Can you work these out from the model? Positions are in its coordinate system, mm. A direction names the side the tool comes from. Give positions to 0.01 mm unless a question says otherwise; leave off trailing zeros. Loops run counter-clockwise (first coordinate to the right, second up) from the corner with the lowest first, then second, coordinate; pieces in that order, holes last. Notation, with made-up numbers: (38, -31.75) - (63, -31.75) arc R34 ccw to (63, 3.25) - close; hole circle Ø5 at (33.25, 11). An arc over 180 degrees is marked (long way). Answer as a JSON object with one key per item and string values. Group by question number.
Item 1: Suppose I cut it at A-A on x = 7.9. Write out the boundary of the cut face in (y, z), and give its area (3 significant figures).
Item 2: Suppose I cut it at C-C on z = -13.5. Write out the boundary of the cut face in (x, y), and give its area (3 significant figures).
Item 3: Suppose I cut it at B-B on y = 1.25. Count the separate pieces of the cut face and the enclosed holes in it, and give its area (3 significant figures).
Item 4: Which directions (+Z, -Z, +X, -X, +Y, -Y) give clear straight access to the entire face, cutting with the end or side of a thin tool? Please do faces 1 (the flat face through (-0.4, 2, -5.1)), 2 (the flat face through (16, 2, -5)), 3 (the cylindrical face through (1.77, 3.99, -2.79)), 4 (the flat face through (-5, 1, -7.4)), 5 (the flat face through (20, 1, -7.4)).
Item 5: Please list where these lines run through material, in increasing order: L1, parallel to X at y = 2.6, z = -3.9; L2, parallel to Z at x = 11.9, y = 2.85; L3, parallel to X at y = 3.3, z = -3.9.
Item 6: Thinking about a two-plate mould opening in Z: for faces 6 (the flat face through (8, 2, -15.8)), 7 (the flat face through (3, 1, -8.6)), 8 (the flat face through (12, 4.8, -4)), which applies, pulls with the +Z half, pulls with the -Z half, needs draft (parallel to the pull), parting line crosses it, or undercut?
Item 7: Will these pins go through, and if not, where does the flat tip stop? pin 1 (4 mm diameter, centred on x = 12, z = -4.5, fed in from -Y); pin 2 (1 mm diameter, centred on x = 0.5, z = -12, fed in from +Y); pin 3 (0.8 mm diameter, centred on x = -5.5, y = 1.5, fed in from +Z).
Item 8: Suppose I cut it at D-D on x = 11.9. Write out the boundary of the cut face in (y, z).
from build123d import *

# Parameters (mm, degrees)
SKETCH1_W                = 15.8
SKETCH1_H                = 3.2
BOSS_EXTRUDE1_DEPTH      = 15.8
SKETCH2_R                = 2.4
BOSS_EXTRUDE2_DEPTH      = 1.6
LPATTERN1_COUNT          = 2
LPATTERN1_PITCH          = 8
LPATTERN1_COUNT_DIR2     = 4
LPATTERN1_PITCH_DIR2     = 8
SHELL1_T                 = -1.2
SKETCH4_R                = 3.25
SKETCH4_R_2              = 2.4
BOSS_EXTRUDE3_DEPTH      = 1.8
BOSS_EXTRUDE4_REACH      = 24.042
BOSS_EXTRUDE4_END_RADIUS = 3.25
SKETCH6_W                = 1.1
SKETCH6_H                = 2
MIRROR1_DEPTH            = 2
BOSS_EXTRUDE6_DEPTH      = 2
BOSS_EXTRUDE7_START      = -0.3
SKETCH9_R                = 2
BOSS_EXTRUDE7_DEPTH      = 1
SKETCH10_R               = 1.55
BOSS_EXTRUDE8_DEPTH      = 5
CUT_EXTRUDE1_START       = -3
CUT_EXTRUDE1_DEPTH       = 3
FILLET1_R                = 0.5
FILLET1_OF_MIRROR2_R     = 0.5


# Read off the part's stored shape, not the designer's step: Mirror1
with BuildPart() as part:
    # Sketch1 → Boss-Extrude1 (new body)
    with BuildSketch(Plane.XY):
        with Locations((7.9, 1.6)):
            Rectangle(SKETCH1_W, SKETCH1_H)
    extrude(amount=-BOSS_EXTRUDE1_DEPTH)

    # Sketch2 → Boss-Extrude2 (add)
    with BuildSketch(Plane(origin=(0, 3.2, 0), x_dir=(1, 0, 0), z_dir=(0, 1, 0))):
        with Locations(Location((3.9, 3.9, 0), (0, 0, 270))):
            Circle(SKETCH2_R)
    boss_extrude2 = extrude(amount=BOSS_EXTRUDE2_DEPTH)

    # LPattern1: Boss-Extrude2 2 × 4, 4 skipped
    with Locations(*[(j * LPATTERN1_PITCH_DIR2, 0, -i * LPATTERN1_PITCH) for i in range(LPATTERN1_COUNT) for j in range(LPATTERN1_COUNT_DIR2) if (i, j) not in ((0, 0), (0, 2), (0, 3), (1, 2), (1, 3))]):
        add(boss_extrude2)

    # Shell1
    shell1_openings = [part.faces().sort_by_distance(p)[0] for p in [
        (7.9, 0, -7.9),
    ]]
    offset(amount=SHELL1_T, openings=shell1_openings, kind=Kind.INTERSECTION)

    # Sketch4 → Boss-Extrude3 (add)
    with BuildSketch(Plane.XZ.offset(-2)):
        with Locations(Location((7.9, -7.9, 0), (0, 0, 90))):
            Circle(SKETCH4_R)
        with Locations(Location((7.9, -7.9, 0), (0, 0, 270))):
            Circle(SKETCH4_R_2, mode=Mode.SUBTRACT)
    extrude(amount=BOSS_EXTRUDE3_DEPTH)

    # Boss-Extrude4: up to this cylinder (the profile starts outside it)
    boss_extrude4_end = Plane(origin=(7.9, 1, -7.9), z_dir=(0, 1, 0)) * Cylinder(BOSS_EXTRUDE4_END_RADIUS, 55.584, mode=Mode.PRIVATE)
    # Sketch6 → Boss-Extrude4 (add, up to the surface)
    with BuildSketch(Plane.ZY.offset(-14.6), mode=Mode.PRIVATE) as boss_extrude4_sk1:
        with Locations((-8.05, 1)):
            Rectangle(SKETCH6_W, SKETCH6_H)
    boss_extrude4_tool1 = extrude(boss_extrude4_sk1.sketch, amount=BOSS_EXTRUDE4_REACH, mode=Mode.PRIVATE) - boss_extrude4_end
    add(boss_extrude4_tool1.solids().sort_by_distance((14.6, 1, -8.05))[0])

    # Mirror1 outline → Mirror1 (add)
    with BuildSketch(Plane(origin=(0, 0, 0), x_dir=(1, 0, 0), z_dir=(0, 1, 0))):
        with BuildLine():
            Line((1.2, 8.6), (1.2, 7.5))
            Line((1.2, 7.5), (4.674709315, 7.5))
            ThreePointArc((4.674709315, 7.5), (4.653565784, 8.052200126), (4.726279785, 8.6))
            Line((4.726279785, 8.6), (1.2, 8.6))
        make_face()
    extrude(amount=MIRROR1_DEPTH)

    # Sketch8 → Boss-Extrude6 (add)
    with BuildSketch(Plane(origin=(0, 0, 0), x_dir=(-1, 0, 0), z_dir=(0, -1, 0))):
        Polygon((1, 10.4), (0, 12.15), (0, 3.65), (1, 5.4), (1, 6.4), (0.3, 6.4), (0.3, 9.4), (1, 9.4), align=None)
    boss_extrude6 = extrude(amount=-BOSS_EXTRUDE6_DEPTH)

    # Sketch9 → Boss-Extrude7 (add)
    with BuildSketch(Plane.ZY.offset(0.3).offset(BOSS_EXTRUDE7_START)):
        with Locations((-7.9, 1.2)):
            Circle(SKETCH9_R)
    boss_extrude7 = extrude(amount=BOSS_EXTRUDE7_DEPTH)

    # Sketch10 → Boss-Extrude8 (add)
    with BuildSketch(Plane.ZY.offset(1)):
        with Locations((-7.9, 1.25)):
            Circle(SKETCH10_R)
    boss_extrude8 = extrude(amount=BOSS_EXTRUDE8_DEPTH)

    # Sketch11 → Cut-Extrude1 (cut)
    with BuildSketch(Plane.ZY.offset(6).offset(CUT_EXTRUDE1_START)):
        with BuildLine():
            Line((-8.4, 2.717140075), (-8.4, -0.217140075))
            ThreePointArc((-8.4, -0.217140075), (-7.9, -0.3), (-7.4, -0.217140075))
            Line((-7.4, -0.217140075), (-7.4, 2.717140075))
            ThreePointArc((-7.4, 2.717140075), (-7.9, 2.8), (-8.4, 2.717140075))
        make_face()
    cut_extrude1 = extrude(amount=CUT_EXTRUDE1_DEPTH, mode=Mode.SUBTRACT)

    # Fillet1
    fillet1_edges = [part.edges().sort_by_distance(p)[0] for p in [
        (-3, 1.25, -8.4),
        (-3, 1.25, -7.4),
    ]]
    fillet(fillet1_edges, radius=FILLET1_R - 0.0001)  # a hair under: the kernel refuses the full size

    # Mirror2: Boss-Extrude6, Boss-Extrude7, Boss-Extrude8, Cut-Extrude1 across plane
    add(boss_extrude6.mirror(Plane(origin=(7.8, 0, 0), x_dir=(0, 0, 1), z_dir=(1, 0, 0))))
    add(boss_extrude7.mirror(Plane(origin=(7.8, 0, 0), x_dir=(0, 0, 1), z_dir=(1, 0, 0))))
    add(boss_extrude8.mirror(Plane(origin=(7.8, 0, 0), x_dir=(0, 0, 1), z_dir=(1, 0, 0))))
    add(cut_extrude1.mirror(Plane(origin=(7.8, 0, 0), x_dir=(0, 0, 1), z_dir=(1, 0, 0))), mode=Mode.SUBTRACT)

    # Fillet1 of Mirror2
    fillet1_of_mirror2_edges = [part.edges().sort_by_distance(p)[0] for p in [
        (18.6, 1.25, -8.4),
        (18.6, 1.25, -7.4),
    ]]
    fillet(fillet1_of_mirror2_edges, radius=FILLET1_OF_MIRROR2_R - 0.0001)  # a hair under: the kernel refuses the full size


solid = part.part
Worked out:
{
 "1": {"outline": "(0, -15.8) - (3.2, -15.8) - (3.2, 0) - (0, 0) - (0, -1.2) - (2, -1.2) - (2, -4.65) - (0.2, -4.65) - (0.2, -5.5) - (2, -5.5) - (2, -10.3) - (0.2, -10.3) - (0.2, -11.15) - (2, -11.15) - (2, -14.6) - (0, -14.6) - close", "area": "26.8 mm2"},
 "2": {"outline": "(0, 0) - (1.2, 0) - (1.2, 2) - (14.6, 2) - (14.6, 0) - (15.8, 0) - (15.8, 3.2) - (13.69, 3.2) - (13.69, 4.8) - (10.11, 4.8) - (10.11, 3.2) - (5.69, 3.2) - (5.69, 4.8) - (2.11, 4.8) - (2.11, 3.2) - (0, 3.2) - close", "area": "35.2 mm2"},
 "3": {"separate pieces": "1", "enclosed holes": "3", "area": "130 mm2"},
 "4": {"face 1": "+Z, -X, +Y", "face 2": "+Z, +X, +Y", "face 3": "+Y", "face 4": "-X, +Y, -Y", "face 5": "+X, +Y, -Y"},
 "5": {"L1": "x = 0 to 2.7, 5.1 to 10.7, 13.1 to 15.8", "L2": "z = -15.8 to -13.1, -10.7 to -5.1, -2.7 to 0", "L3": "x = 1.5 to 2.7, 5.1 to 6.3, 9.5 to 10.7, 13.1 to 14.3"},
 "6": {"face 6": "pulls with the -Z half", "face 7": "undercut", "face 8": "needs draft"},
 "7": {"pin 1": "stops at y = 2", "pin 2": "stops at y = 3.2", "pin 3": "stops at z = -6.35"},
 "8": {"outline": "(0, -15.8) - (3.2, -15.8) - (3.2, -14.3) - (4.8, -14.3) - (4.8, -9.5) - (3.2, -9.5) - (3.2, -6.3) - (4.8, -6.3) - (4.8, -1.5) - (3.2, -1.5) - (3.2, 0) - (0, 0) - (0, -1.2) - (2, -1.2) - (2, -2.7) - (3.6, -2.7) - (3.6, -5.1) - (2, -5.1) - (2, -7.5) - (0, -7.5) - (0, -8.6) - (2, -8.6) - (2, -10.7) - (3.6, -10.7) - (3.6, -13.1) - (2, -13.1) - (2, -14.6) - (0, -14.6) - close"}
}
